from build123d import *

# Parameters (mm, degrees)
F1_DEPTH = 45
F2_R     = 2.1
F3_DEPTH = 12
F4_SIZE  = 0.99999


# Not quite as in the source:
# - a fillet or chamfer is up to 0.001 mm smaller than in the source, because OpenCascade refuses the exact size


with BuildPart() as f1:
    # F0 (on Front) → F1 (new body)
    with BuildSketch(Plane.XZ):
        with BuildLine():
            Line((88.0538091608, -30.5978502929), (75.0538091608, -30.5978502929))
            Line((75.0538091608, -30.5978502929), (75.0538091608, -39.5978502929))
            Line((75.0538091608, -39.5978502929), (76.0538091608, -39.5978502929))
            Line((76.0538091608, -39.5978502929), (76.0538091608, -63.5978502929))
            Line((76.0538091608, -63.5978502929), (86.6455139554, -63.5978502929))
            Line((86.6455139554, -63.5978502929), (92.4115082833, -56.7262058379))
            ThreePointArc((92.4115082833, -56.7262058379), (97.5538091608, -42.5978502929), (102.6961100382, -56.7262058379))
            Line((102.6961100382, -56.7262058379), (108.4621043661, -63.5978502929))
            Line((108.4621043661, -63.5978502929), (119.0538091608, -63.5978502929))
            Line((119.0538091608, -63.5978502929), (119.0538091608, -39.5978502929))
            Line((119.0538091608, -39.5978502929), (120.0538091608, -39.5978502929))
            Line((120.0538091608, -39.5978502929), (120.0538091608, -30.5978502929))
            Line((120.0538091608, -30.5978502929), (107.0538091608, -30.5978502929))
            Line((107.0538091608, -30.5978502929), (107.0538091608, -31.5978502929))
            Line((107.0538091608, -31.5978502929), (88.0538091608, -31.5978502929))
            Line((88.0538091608, -31.5978502929), (88.0538091608, -30.5978502929))
        make_face()
    extrude(amount=F1_DEPTH)

    # F2 (on face) → F3 (cut)
    with BuildSketch(Plane.XY.offset(-30.5978502929)):
        with Locations((81.5538091608, -7.5)):
            Circle(F2_R)
        with Locations((81.5538091608, -37.5)):
            Circle(F2_R)
        with Locations((113.5538091608, -7.5)):
            Circle(F2_R)
        with Locations((113.5538091608, -37.5)):
            Circle(F2_R)
    extrude(amount=-F3_DEPTH, mode=Mode.SUBTRACT)

    # F4 (size 1 in the source; OpenCascade refuses exactly that, so slightly less here)
    f4_edges = [f1.edges().sort_by_distance(p)[0] for p in [
        (88.053809, -22.5, -30.59785),
        (107.053809, -22.5, -30.59785),
        (75.053809, -22.5, -30.59785),
        (75.053809, -22.5, -39.59785),
        (120.053809, -22.5, -30.59785),
        (120.053809, -22.5, -39.59785),
        (76.053809, -22.5, -63.59785),
        (119.053809, -22.5, -63.59785),
    ]]
    chamfer(f4_edges, length=F4_SIZE)


solid = f1.part
Check sheet for the modelled part. Datum: model origin and axes. Units: mm. A direction names the side the tool comes from. Coordinates: 2 decimals unless noted, no trailing zeros. Write each loop counter-clockwise with the first axis right and the second up, starting at its lowest first coordinate (ties: lowest second). Pieces come first, ordered by that corner, then holes.
Item 1: Scan lines: probe 1 along X at (y, z) = (-9, -62); probe 2 along X at (y, z) = (-18, -48); probe 3 along X at (y, z) = (-37, -37). Record each from-to range of solid material in increasing order.
Numbers:
probe 1: x = 76.05 to 87.99, 107.12 to 119.05
probe 2: x = 76.05 to 89.99, 105.12 to 119.05
probe 3: x = 75.05 to 79.51, 83.59 to 111.51, 115.59 to 120.05
Item 2: Depth check by flat-ended pin: pin 1 Ø5 at (y, z) = (-31, -55) entering from +X; pin 2 Ø1.5 at (x, y) = (96.5, -10) entering from +Z; pin 3 Ø2 at (x, y) = (95.5, -12) entering from -Z. Enter the tip coordinate at first touch or a pass-through.
Numbers:
pin 1: stops at x = 119.05
pin 2: stops at z = -31.6
pin 3: stops at z = -43.2
Item 3: Mould release check, pull along Y, two halves, no side actions. Record for faces 6 (the face through (92, -45, -43)), 7 (the face through (82, -7, -42.598)), 8 (the face through (113, -22, -63.598)), 9 (the face through (114, -37, -42.598)): released by +Y, released by -Y, zero draft, split by the parting line, or undercut.
Numbers:
face 6: released by -Y
face 7: undercut
face 8: zero draft
face 9: undercut
Item 4: Cross-section at A-A on z = -42. Record the boundary of the cut face in (x, y).
Numbers:
outline: (76.05, -45) - (119.05, -45) - (119.05, 0) - (76.05, 0) - close; hole circle Ø4.2 at (81.55, -37.5); hole circle Ø4.2 at (81.55, -7.5); hole circle Ø4.2 at (113.55, -37.5); hole circle Ø4.2 at (113.55, -7.5)
Item 5: Cross-section at C-C on x = 103.5. Record the boundary of the cut face in (y, z), then the cut area to 3 significant figures.
Numbers:
outline: (-45, -57.68) - (0, -57.68) - (0, -55.95) - (-45, -55.95) - close; (-45, -45.25) - (0, -45.25) - (0, -31.6) - (-45, -31.6) - close
area: 692 mm2
Item 6: Access from +Z, -Z, +X, -X, +Y, -Y to the whole of each face (thin tool, end or side, straight path). Record for faces 1 (the face through (82, -37, -42.598)), 2 (the face through (119.054, -22, -51)), 3 (the face through (105.539, -22.185, -60.114)), 4 (the face through (76.054, -22, -51)), 5 (the face through (98, -22, -31.598)).
Numbers:
face 1: +Z
face 2: -Z, +X, +Y, -Y
face 3: -Z, +Y, -Y
face 4: -Z, -X, +Y, -Y
face 5: +Z, +Y, -Y
Item 7: Cross-section at D-D on z = -36. Record the boundary of the cut face in (x, y), then the cut area to 3 significant figures.
Numbers:
outline: (75.05, -45) - (120.05, -45) - (120.05, 0) - (75.05, 0) - close; hole circle Ø4.2 at (81.55, -37.5); hole circle Ø4.2 at (81.55, -7.5); hole circle Ø4.2 at (113.55, -37.5); hole circle Ø4.2 at (113.55, -7.5)
area: 1,970 mm2
